Build history of the part. All positions in model axes, mm. Face numbers are marked on the shaded views. A direction names the side the tool comes from. Round coordinates to 2 decimals unless told otherwise and drop trailing zeros. Order: outer loops, then holes, each group sorted by start corner. A loop starts at its lowest first (then second) coordinate and runs counter-clockwise, first axis right, second up. Notation, with made-up numbers: (-22.5, 74.25) -> (4.5, 74.25) arc R22 cw to (4.5, 109.25) -> close; hole circle Ø9 at (-24, 39.25). An arc over 180 degrees is marked (long way). Answer as a JSON object with one key per item and string values.
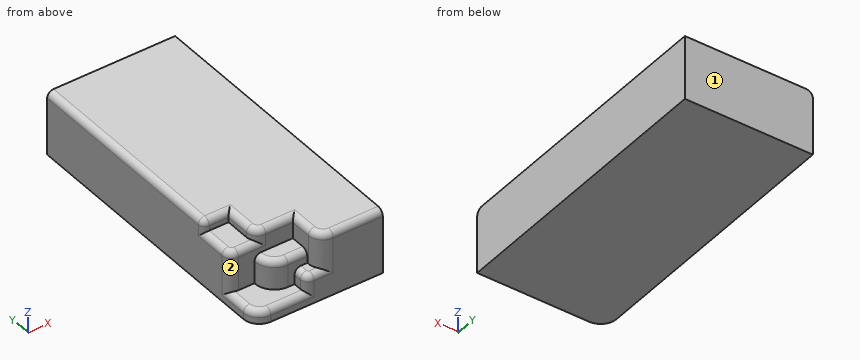
from build123d import *

# Parameters (mm, degrees)
F1_DEPTH = 80
F2_W     = 80
F2_H     = 225
F3_DEPTH = 320
F4_DEPTH = 250
F2_H_2   = 125
F5_DEPTH = 180
F6_DEPTH = 100
F7_R     = 40


with BuildPart() as f1:
    # F0 (on Top) → F1 (new body)
    with BuildSketch(Plane.XY):
        with BuildLine():
            ThreePointArc((-400, -800), (-370.7106781187, -870.7106781187), (-300, -900))
            Line((-300, -900), (400, -900))
            Line((400, -900), (400, 900))
            Line((400, 900), (-400, 900))
            Line((-400, 900), (-400, -800))
        make_face()
    extrude(amount=F1_DEPTH)

    # F2 (on face) → F3 (join)
    with BuildSketch(Plane.XY.offset(80)):
        with BuildLine():
            Line((400, -900), (400, 900))
            Line((400, 900), (-400, 900))
            Line((-400, 900), (-400, 0))
            Line((-400, 0), (0, 0))
            Line((0, 0), (0, -450))
            Line((0, -450), (0, -675))
            Line((0, -675), (0, -800))
            Line((0, -800), (0, -810))
            ThreePointArc((0, -810), (26.3603896932, -873.6396103068), (90, -900))
            Line((90, -900), (122.6464435458, -900))
            Line((122.6464435458, -900), (400, -900))
        make_face()
        with BuildLine():
            Line((0, 0), (-400, 0))
            Line((-400, 0), (-400, -410))
            ThreePointArc((-400, -410), (-388.2842712475, -438.2842712475), (-360, -450))
            Line((-360, -450), (-240, -450))
            Line((-240, -450), (-80, -450))
            Line((-80, -450), (0, -450))
            Line((0, -450), (0, 0))
        make_face()
        with Locations((-40, -562.5)):
            Rectangle(F2_W, F2_H)
        with BuildLine():
            Line((-80, -450), (-240, -450))
            Line((-240, -450), (-240, -605))
            ThreePointArc((-240, -605), (-219.4974746831, -654.4974746831), (-170, -675))
            Line((-170, -675), (-80, -675))
            Line((-80, -675), (-80, -450))
        make_face()
    extrude(amount=F3_DEPTH)

    # F2 (on face) → F4 (join)
    with BuildSketch(Plane.XY.offset(80)):
        with BuildLine():
            ThreePointArc((-360, -450), (-388.2842712475, -438.2842712475), (-400, -410))
            Line((-400, -410), (-400, -450))
            Line((-400, -450), (-400, -615))
            ThreePointArc((-400, -615), (-382.4264068712, -657.4264068712), (-340, -675))
            Line((-340, -675), (-240, -675))
            Line((-240, -675), (-240, -605))
            Line((-240, -605), (-240, -450))
            Line((-240, -450), (-360, -450))
        make_face()
        with BuildLine():
            ThreePointArc((-170, -675), (-219.4974746831, -654.4974746831), (-240, -605))
            Line((-240, -605), (-240, -675))
            Line((-240, -675), (-170, -675))
        make_face()
    extrude(amount=F4_DEPTH)

    # F2 (on face) → F5 (join)
    with BuildSketch(Plane.XY.offset(80)):
        with BuildLine():
            Line((-80, -800), (-80, -675))
            Line((-80, -675), (-170, -675))
            Line((-170, -675), (-240, -675))
            Line((-240, -675), (-240, -680))
            ThreePointArc((-240, -680), (-204.8528137424, -764.8528137424), (-120, -800))
            Line((-120, -800), (-80, -800))
        make_face()
        with Locations((-40, -562.5)):
            Rectangle(F2_W, F2_H)
        with Locations((-40, -737.5)):
            Rectangle(F2_W, F2_H_2)
        with BuildLine():
            ThreePointArc((-170, -675), (-219.4974746831, -654.4974746831), (-240, -605))
            Line((-240, -605), (-240, -675))
            Line((-240, -675), (-170, -675))
        make_face()
    extrude(amount=F5_DEPTH)

    # F2 (on face) → F6 (join)
    with BuildSketch(Plane.XY.offset(80)):
        with Locations((-40, -562.5)):
            Rectangle(F2_W, F2_H)
        with Locations((-40, -737.5)):
            Rectangle(F2_W, F2_H_2)
        with BuildLine():
            Line((-30, -900), (0, -900))
            Line((0, -900), (0, -810))
            Line((0, -810), (0, -800))
            Line((0, -800), (-80, -800))
            Line((-80, -800), (-80, -850))
            ThreePointArc((-80, -850), (-65.3553390593, -885.3553390593), (-30, -900))
        make_face()
        with BuildLine():
            Line((0, -900), (90, -900))
            ThreePointArc((90, -900), (26.3603896932, -873.6396103068), (0, -810))
            Line((0, -810), (0, -900))
        make_face()
    extrude(amount=F6_DEPTH)

    # F7
    f7_edges = [f1.edges().sort_by_distance(p)[0] for p in [
        (-219.497475, -654.497475, 400),
        (26.36039, -873.63961, 400),
        (-300, -450, 400),
        (-382.426407, -657.426407, 330),
        (-204.852814, -764.852814, 260),
        (-65.355339, -885.355339, 180),
        (-370.710678, -870.710678, 80),
    ]]
    fillet(f7_edges, radius=F7_R)


solid = f1.part
1) Probe L1, parallel to Y at x = -112.5, z = 194; L2, parallel to X at y = -807.5, z = 87.5; L3, parallel to Y at x = -281.5, z = 95. List the from-to ranges inside material, lowest first. Write a range as from..to.
Checked values:
{"L1": "y = -800..900", "L2": "x = -80..400", "L3": "y = -675..900"}
2) Flat gauge pins, fed straight in: pin 1 Ø3 at (x, z) = (-245.5, 332.5) entering from -Y; pin 2 Ø15 at (y, z) = (-832.5, 100) entering from -X; pin 3 Ø24 at (y, z) = (-549.5, 349) entering from -X. Where does each tip first touch, or does it go through?
Checked values:
{"pin 1": "stops at y = -450", "pin 2": "stops at x = -80", "pin 3": "stops at x = -240"}
3) Cut at A-A, the plane z = 201. Give the cut face in (x, y).
Checked values:
{"outline": "(-400, -615) arc R60 ccw to (-340, -675) -> (-240, -675) -> (-240, -680) arc R120 ccw to (-120, -800) -> (0, -800) -> (0, -810) arc R90 ccw to (90, -900) -> (400, -900) -> (400, 900) -> (-400, 900) -> close"}
4) Cut at B-B, the plane x = -266. Give the cut face in (y, z).
Checked values:
{"outline": "(-900, 0) -> (900, 0) -> (900, 400) -> (-410, 400) arc R40 ccw to (-450, 360) -> (-450, 330) -> (-635, 330) arc R40 ccw to (-675, 290) -> (-675, 80) -> (-860, 80) arc R40 ccw to (-900, 40) -> close"}
5) Which spindle directions (+Z, -Z, +X, -X, +Y, -Y) get a long thin tool onto all of the face, cutting with end or side? Do the marked faces 1 and 2. Say none if no direction does.
Checked values:
{"face 1": "+Z, -Z, +X, -X, +Y", "face 2": "+Z, -X, -Y"}
